Input: dimensioned drawing with shaded views. Units: mm. Origin: part minimum x, y, z. A direction names the side the tool comes from. Give positions to 0.01 mm unless a question says otherwise; leave off trailing zeros. Write each loop counter-clockwise with the first axis right and the second up, starting at its lowest first coordinate (ties: lowest second). Pieces come first, ordered by that corner, then holes.
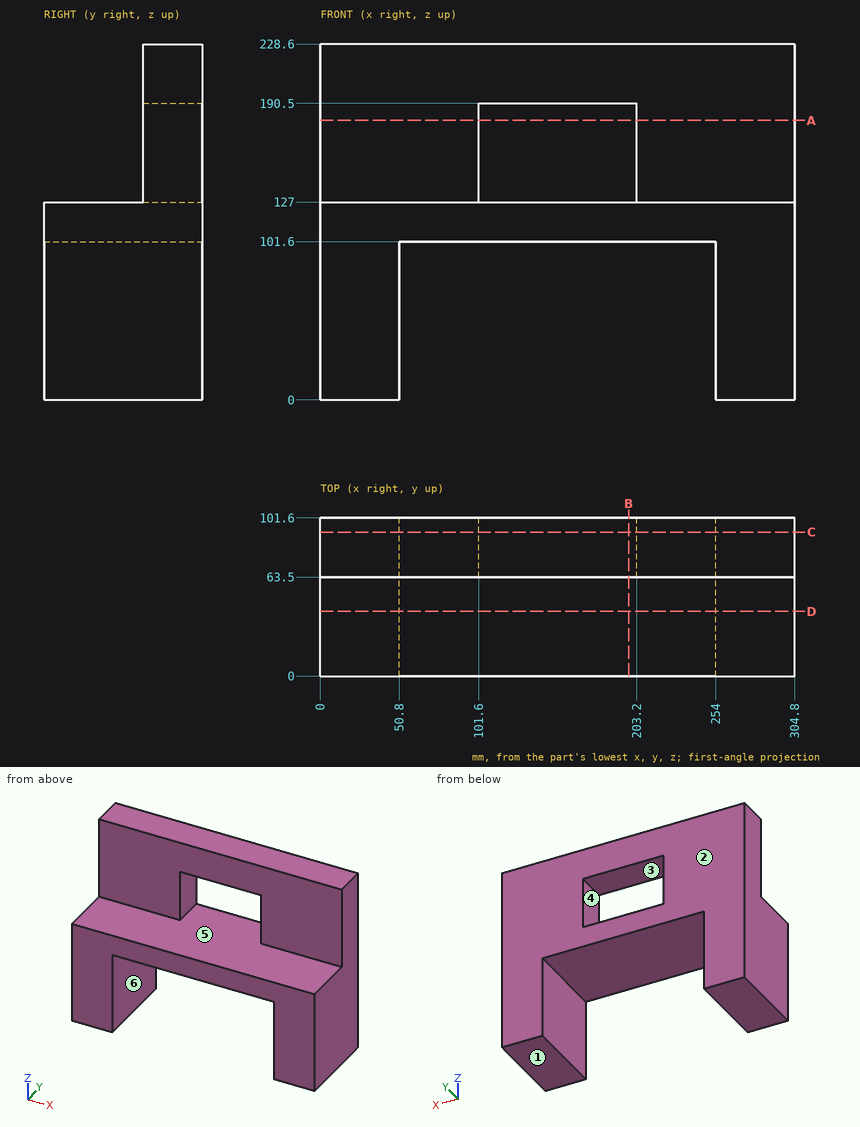
Item 1: Reachability of the marked faces 4, 5 and 6 from +Z, -Z, +X, -X, +Y, -Y: full face, straight path, thin tool, end or side. Return the list, or none.
Found:
face 4: +Y, -Y
face 5: -Y
face 6: -Z, +Y, -Y
Item 2: Line query: L1, parallel to X at y = 49, z = 27.5; L2, parallel to X at y = 72, z = 160; L3, parallel to Z at x = 141, y = 70.5. Output: solid intervals per line, ascending.
Found:
L1: x = 0 to 50.8, 254 to 304.8
L2: x = 0 to 101.6, 203.2 to 304.8
L3: z = 101.6 to 127, 190.5 to 228.6
Item 3: Section B-B, the plane x = 198. Return the cut outline in (y, z).
Found:
outline: (0, 101.6) - (101.6, 101.6) - (101.6, 127) - (0, 127) - close; (63.5, 190.5) - (101.6, 190.5) - (101.6, 228.6) - (63.5, 228.6) - close
Item 4: Section C-C, the plane y = 92.5. Return the cut outline in (x, z).
Found:
outline: (0, 0) - (50.8, 0) - (50.8, 101.6) - (254, 101.6) - (254, 0) - (304.8, 0) - (304.8, 228.6) - (0, 228.6) - close; hole (101.6, 127) - (203.2, 127) - (203.2, 190.5) - (101.6, 190.5) - close
Item 5: Pull-direction query (Z, two-part tool) for the marked faces 1, 2 and 3; classes: +Z half, -Z half, draft (parallel to the pull), parting line (faces both ways), or undercut.
Found:
face 1: -Z half
face 2: draft
face 3: undercut
Item 6: Pin query (flat end, axial travel): pin 1 Ø12 at (x, z) = (203.5, 108) entering from -Y; pin 2 Ø5 at (x, y) = (226.5, 24.5) entering from -Z; pin 3 Ø1 at (x, y) = (93.5, 38.5) entering from +Z; pin 4 Ø4 at (x, z) = (263.5, 177) entering from -Y. Return the tip coordinate at first contact, or that it passes through.
Found:
pin 1: stops at y = 0
pin 2: stops at z = 101.6
pin 3: stops at z = 127
pin 4: stops at y = 63.5
Item 7: Section D-D, the plane y = 41.5. Return the cut outline in (x, z).
Found:
outline: (0, 0) - (50.8, 0) - (50.8, 101.6) - (254, 101.6) - (254, 0) - (304.8, 0) - (304.8, 127) - (0, 127) - close
Item 8: Section A-A, the plane z = 179.5. Return the cut outline in (x, y), plus the area to 3 significant figures.
Found:
outline: (0, 63.5) - (101.6, 63.5) - (101.6, 101.6) - (0, 101.6) - close; (203.2, 63.5) - (304.8, 63.5) - (304.8, 101.6) - (203.2, 101.6) - close
area: 7,740 mm2
